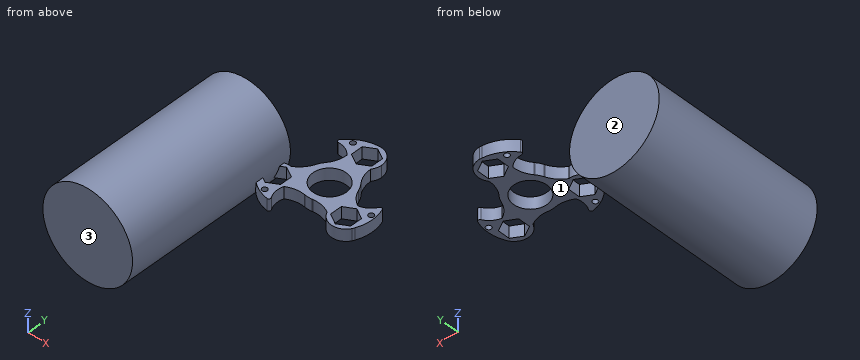
from build123d import *

# Parameters (mm, degrees)
F0_R     = 1.78928
F0_R_2   = 11.43
F1_DEPTH = 8.128
F2_R     = 1.27
F3_R     = 30.929844
F4_DEPTH = 118.11


with BuildPart() as f1:
    # F0 (on Top) → F1 (new body)
    with BuildSketch(Plane.XY):
        with BuildLine():
            ThreePointArc((12.152307, 10.214552), (9.141542, 15.705526), (8.1629, 21.890813))
            ThreePointArc((8.1629, 21.890813), (0, 17.78), (-8.1629, 21.890813))
            ThreePointArc((-8.1629, 21.890813), (-9.120339, 15.730112), (-12.113273, 10.260811))
            ThreePointArc((-12.113273, 10.260811), (0.030263, 15.874971), (12.152307, 10.214552))
        make_face()
        with BuildLine():
            ThreePointArc((10.16, 27.94), (7.184205, 35.124205), (0, 38.1))
            ThreePointArc((0, 38.1), (-0.774338, 38.052294), (-1.546912, 37.981547))
            ThreePointArc((-1.546912, 37.981547), (-9.396704, 31.80362), (-8.1629, 21.890813))
            ThreePointArc((-8.1629, 21.890813), (0, 17.78), (8.1629, 21.890813))
            ThreePointArc((8.1629, 21.890813), (9.647815, 24.754836), (10.16, 27.94))
        make_face()
        Polygon((-6.985, 31.972792), (0, 36.005583), (6.985, 31.972792), (6.985, 23.907208), (0, 19.874417), (-6.985, 23.907208), align=None, mode=Mode.SUBTRACT)
        with BuildLine():
            ThreePointArc((-8.1629, 21.890813), (-9.396704, 31.80362), (-1.546912, 37.981547))
            ThreePointArc((-1.546912, 37.981547), (-12.612928, 34.15479), (-20.884238, 25.867077))
            ThreePointArc((-20.884238, 25.867077), (-13.967457, 25.658122), (-8.1629, 21.890813))
        make_face()
        with Locations((-12.453423, 30.944496)):
            Circle(F0_R, mode=Mode.SUBTRACT)
        with BuildLine():
            ThreePointArc((2.348846, -15.700272), (2.559176, -15.664647), (2.769908, -15.631482))
            ThreePointArc((2.769908, -15.631482), (12.165277, -10.199101), (15.875, 0))
            ThreePointArc((15.875, 0), (15.640204, 2.720232), (14.942759, 5.359997))
            ThreePointArc((14.942759, 5.359997), (14.855473, 5.587409), (14.771257, 5.815976))
            ThreePointArc((14.771257, 5.815976), (13.748153, 7.9375), (12.422412, 9.884296))
            ThreePointArc((12.422412, 9.884296), (12.286395, 10.048635), (12.152307, 10.214552))
            ThreePointArc((12.152307, 10.214552), (0.030263, 15.874971), (-12.113273, 10.260811))
            ThreePointArc((-12.113273, 10.260811), (-12.266574, 10.071512), (-12.422412, 9.884296))
            ThreePointArc((-12.422412, 9.884296), (-13.748153, 7.9375), (-14.771257, 5.815976))
            ThreePointArc((-14.771257, 5.815976), (-14.845571, 5.616012), (-14.922215, 5.41693))
            ThreePointArc((-14.922215, 5.41693), (-13.76326, -7.911277), (-2.829486, -15.620808))
            ThreePointArc((-2.829486, -15.620808), (-2.588898, -15.658921), (-2.348846, -15.700272))
            ThreePointArc((-2.348846, -15.700272), (0, -15.875), (2.348846, -15.700272))
        make_face()
        Circle(F0_R_2, mode=Mode.SUBTRACT)
        with BuildLine():
            ThreePointArc((-23.03945, -3.876128), (-32.691442, -8.39633), (-32.995568, -19.05))
            ThreePointArc((-32.995568, -19.05), (-32.567084, -19.696744), (-32.119528, -20.330439))
            ThreePointArc((-32.119528, -20.330439), (-22.844391, -24.039594), (-14.87655, -18.014685))
            ThreePointArc((-14.87655, -18.014685), (-14.248915, -16.035474), (-14.03675, -13.97))
            ThreePointArc((-14.03675, -13.97), (-16.614409, -7.207329), (-23.03945, -3.876128))
        make_face()
        Polygon((-17.21175, -9.937208), (-17.21175, -18.002792), (-24.19675, -22.035583), (-31.18175, -18.002792), (-31.18175, -9.937208), (-24.19675, -5.904417), align=None, mode=Mode.SUBTRACT)
        with BuildLine():
            ThreePointArc((-14.922215, 5.41693), (-18.172156, 0.064044), (-23.03945, -3.876128))
            ThreePointArc((-23.03945, -3.876128), (-16.614409, -7.207329), (-14.03675, -13.97))
            ThreePointArc((-14.03675, -13.97), (-14.248915, -16.035474), (-14.87655, -18.014685))
            ThreePointArc((-14.87655, -18.014685), (-9.062508, -15.763501), (-2.829486, -15.620808))
            ThreePointArc((-2.829486, -15.620808), (-13.76326, -7.911277), (-14.922215, 5.41693))
        make_face()
        with BuildLine():
            ThreePointArc((-14.87655, -18.014685), (-22.844391, -24.039594), (-32.119528, -20.330439))
            ThreePointArc((-32.119528, -20.330439), (-23.272452, -28.000511), (-11.959427, -31.019819))
            ThreePointArc((-11.959427, -31.019819), (-15.236857, -24.925234), (-14.87655, -18.014685))
        make_face()
        with Locations((-20.572009, -26.257229)):
            Circle(F0_R, mode=Mode.SUBTRACT)
        with BuildLine():
            ThreePointArc((2.769908, -15.631482), (9.030614, -15.76957), (14.87655, -18.014685))
            ThreePointArc((14.87655, -18.014685), (15.397932, -8.89), (23.03945, -3.876128))
            ThreePointArc((23.03945, -3.876128), (18.182846, 0.033389), (14.942759, 5.359997))
            ThreePointArc((14.942759, 5.359997), (15.640204, 2.720232), (15.875, 0))
            ThreePointArc((15.875, 0), (12.165277, -10.199101), (2.769908, -15.631482))
        make_face()
        with BuildLine():
            ThreePointArc((14.87655, -18.014685), (23.617156, -24.113455), (32.995568, -19.05))
            ThreePointArc((32.995568, -19.05), (33.341423, -18.355551), (33.666441, -17.651108))
            ThreePointArc((33.666441, -17.651108), (34.182681, -15.842637), (34.35675, -13.97))
            ThreePointArc((34.35675, -13.97), (30.95942, -6.38766), (23.03945, -3.876128))
            ThreePointArc((23.03945, -3.876128), (15.397932, -8.89), (14.87655, -18.014685))
        make_face()
        Polygon((17.21175, -9.937208), (24.19675, -5.904417), (31.18175, -9.937208), (31.18175, -18.002792), (24.19675, -22.035583), (17.21175, -18.002792), align=None, mode=Mode.SUBTRACT)
        with BuildLine():
            ThreePointArc((34.35675, -13.97), (34.182681, -15.842637), (33.666441, -17.651108))
            ThreePointArc((33.666441, -17.651108), (35.88538, -6.154279), (32.843664, 5.152742))
            ThreePointArc((32.843664, 5.152742), (29.204314, -0.732888), (23.03945, -3.876128))
            ThreePointArc((23.03945, -3.876128), (30.95942, -6.38766), (34.35675, -13.97))
        make_face()
        with Locations((33.025431, -4.687268)):
            Circle(F0_R, mode=Mode.SUBTRACT)
    extrude(amount=F1_DEPTH)

    # F2
    f2_edges = [f1.edges().sort_by_distance(p)[0] for p in [
        (-20.884238, 25.867077, 4.064),
        (-11.959427, -31.019819, 4.064),
        (32.843664, 5.152742, 4.064),
    ]]
    fillet(f2_edges, radius=F2_R)

    # F3 (on Front) → F4 (join)
    with BuildSketch(Plane.XZ):
        with Locations((-57.932083, 13.224379)):
            Circle(F3_R)
    extrude(amount=F4_DEPTH)


solid = f1.part
Design review of the part built by this model. Coordinates are the model's own, in mm. Face numbers are marked on the shaded views. A direction names the side the tool comes from. Round coordinates to 2 decimals unless told otherwise and drop trailing zeros. Loops run counter-clockwise (first coordinate to the right, second up) from the corner with the lowest first, then second, coordinate; pieces in that order, holes last. Notation, with made-up numbers: (59, 0.25) -> (110, 0.25) arc R27 cw to (110, 30.25) -> close; hole circle Ø7 at (83.5, 57). An arc over 180 degrees is marked (long way). Use one line per item in the form item = value. Start each with the question number.
Q1. We need section C-C on y = -83.5. Give the boundary of the cut face in (x, z).
Q2. Machinability: for the marked faces 1, 2 and 3, which of the approach directions +Z, -Z, +X, -X, +Y, -Y give a long, thin tool a straight path to every point of the face, cutting with its end or side? Answer none if there is none.
Q3. Wall thickness on line 1 along Y through (x, z) = (-59, -5); line 2 along X through (y, z) = (-60, 14); line 3 along Z through (x, y) = (-57, -12.5): over which ranges is each line inside the solid? List them lowest first. Write a range as [from, to].
Q4. We need section D-D on z = 34. Give the boundary of the cut face in (x, y).
Q5. We need section A-A on z = 6. State how many separate pieces and enclosed holes the cut face has, then the cut area to 3 significant figures.
Q6. We need section B-B on z = -2. Give the boundary of the cut face in (x, y).
Q7. For pin 1 Ø4 at (y, z) = (-14, 2.5) entering from +X; pin 2 Ø5.5 at (x, y) = (-20.57, -26.26) entering from +Z; pin 3 Ø9 at (y, z) = (-12, 4) entering from -X, all flat-tipped, find the tip position at first contact; note any pin that passes through.
Calculated:
q1.outline = circle Ø61.86 at (-57.93, 13.22)
q2.face_1 = -Z, +X, +Y, -Y
q2.face_2 = +Z, -Z, -X, +Y
q2.face_3 = +Z, -Z, +X, -X, -Y
q3.line_1 = [-118.11, 0]
q3.line_2 = [-88.85, -27.01]
q3.line_3 = [-17.69, 44.14]
q4.outline = (-80.85, -118.11) -> (-35.02, -118.11) -> (-35.02, 0) -> (-80.85, 0) -> close
q5.separate_pieces = 1
q5.enclosed_holes = 7
q5.area = 8,320 mm²
q6.outline = (-84.86, -118.11) -> (-31.01, -118.11) -> (-31.01, 0) -> (-84.86, 0) -> close
q7.pin_1 = 35.44
q7.pin_2 = 8.13
q7.pin_3 = -88.5
